Autodesk Inventor part; units mm, degrees
ref_plane "YZ Plane" through (0, 0, 0) normal (1, 0, 0) x (0, 1, 0)
ref_plane "XZ Plane" through (0, 0, 0) normal (0, 1, 0) x (-1, 0, 0)
ref_plane "XY Plane" through (0, 0, 0) normal (0, 0, 1) x (1, 0, 0)
sketch "Sketch1" plane through (0, 0, 0) normal (1, 0, 0) x (0, 1, 0)
  line L0 (-9.525, 19.05) -> (-9.525, -19.05)
  line L1 (-9.525, -19.05) -> (9.525, -19.05)
  line L2 (9.525, -19.05) -> (9.525, 19.05)
  line L3 (9.525, 19.05) -> (-9.525, 19.05)
  line L4 (-9.525, 19.05) -> (9.525, -19.05) construction
  line L5 (-9.525, -19.05) -> (9.525, 19.05) construction
  line L6 (-6.35, 15.875) -> (-6.35, -15.875)
  line L7 (-6.35, -15.875) -> (6.35, -15.875)
  line L8 (6.35, -15.875) -> (6.35, 15.875)
  line L9 (6.35, 15.875) -> (-6.35, 15.875)
  line L10 (-6.35, 15.875) -> (6.35, -15.875) construction
  line L11 (-6.35, -15.875) -> (6.35, 15.875) construction
  point P0 (0, 0)
  dimension "d0" = 19.05
  dimension "d1" = 38.1
  dimension "d2" = 3.175
  dimension "d3" = 3.175
extrude "Extrusion1" add sketch "Sketch1" along normal mid plane 558.8
equation "\"d0\" = width"
equation "\"d1\" = height"
equation "\"d2\" = wallThickness"
equation "\"d3\" = wallThickness"
equation "\"d4\" = length"
equation "\"width\" = 19.05"
equation "\"height\" = 38.1"
equation "\"length\" = 558.8"
equation "\"wallThickness\" = 3.175"
properties part number "3_4x1_1_2_alumTubing" material "Aluminum 6061"
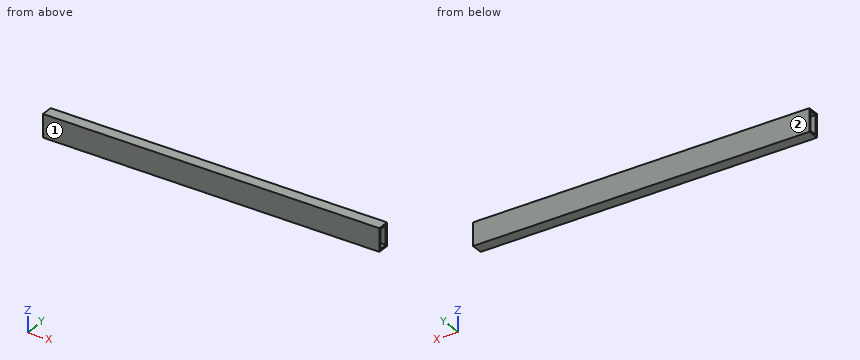
Design review of the part built by this model. Coordinates are the model's own, in mm. Face numbers are marked on the shaded views. Coordinates: 2 decimals unless noted, no trailing zeros. Order: outer loops, then holes, each group sorted by start corner. A loop starts at its lowest first (then second) coordinate and runs counter-clockwise, first axis right, second up. Notation, with made-up numbers: (89.5, 38.5) -> (128.5, 38.5) arc R26 ccw to (128.5, 62.5) -> close; hole circle Ø3 at (74.5, 63). An arc over 180 degrees is marked (long way). One line per item, written item: value. Start each with the question number.
Q1. For probe 1 along Y at (x, z) = (84, -8) (3 decimals); probe 2 along Z at (x, y) = (-41, 5.75) (3 decimals), list the stretches that pass through material, from the lowest coordinate up.
Q2. Take a section at B-B, the plane z = -7.5. State the section outline as (x, y) points (3 decimals), then the cut area to 3 significant figures.
Q3. Mouldability with a two-part tool opening along Y and no side actions: class the marked faces 1 and 2 as pulls with the +Y half, pulls with the -Y half, needs draft (parallel to the pull), parting line crosses it, or undercut.
Q4. Take a section at C-C, the plane x = 240. State the section outline as (y, z) points (3 decimals), then the cut area to 3 significant figures.
Q5. Take a section at A-A, the plane y = 1.25. State the section outline as (x, z) points (3 decimals), then the cut area to 3 significant figures.
Values follow:
1. probe 1: y = -9.525 to -6.35, 6.35 to 9.525
1. probe 2: z = -19.05 to -15.875, 15.875 to 19.05
2. outline: (-279.4, -9.525) -> (279.4, -9.525) -> (279.4, -6.35) -> (-279.4, -6.35) -> close; (-279.4, 6.35) -> (279.4, 6.35) -> (279.4, 9.525) -> (-279.4, 9.525) -> close
2. area: 3,550 mm2
3. face 1: pulls with the -Y half
3. face 2: pulls with the +Y half
4. outline: (-9.525, -19.05) -> (9.525, -19.05) -> (9.525, 19.05) -> (-9.525, 19.05) -> close; hole (-6.35, -15.875) -> (6.35, -15.875) -> (6.35, 15.875) -> (-6.35, 15.875) -> close
4. area: 323 mm2
5. outline: (-279.4, -19.05) -> (279.4, -19.05) -> (279.4, -15.875) -> (-279.4, -15.875) -> close; (-279.4, 15.875) -> (279.4, 15.875) -> (279.4, 19.05) -> (-279.4, 19.05) -> close
5. area: 3,550 mm2
